Can you work these out from the model? Positions are in its coordinate system, mm. A direction names the side the tool comes from. Coordinates: 2 decimals unless noted, no trailing zeros. Loops run counter-clockwise (first coordinate to the right, second up) from the corner with the lowest first, then second, coordinate; pieces in that order, holes last. Notation, with made-up numbers: (23, 10) -> (62, 10) arc R14 cw to (62, 30) -> close; hole circle Ø9 at (88, 11.5). An arc over 180 degrees is marked (long way). Use one line per item in the form item = value. Start each with the question number.
(1) Imagine slicing it at C-C (x = 12.5). List the corners of the cut face in (y, z) for me, plus the area to 3 significant figures.
(2) I need wall thicknesses on line 1 (X direction, y = 21, z = -35); line 2 (Z direction, x = -29, y = -12.5); line 3 (Z direction, x = -39, y = -20.5). Which ranges of each line are inside material? Lowest first, please. Write a range as [from, to].
(3) Thinking about a two-plate mould opening in X: for faces 6 (the cylindrical face through (-43, -22, -39)), 7 (the cylindrical face through (43, -22, -39)), 8 (the flat face through (35, -21, -20)), which applies, released by +X, released by -X, zero draft, split by the parting line, or undercut?
(4) I'm going to push flat-ended pins straight in: pin 1 (4 mm diameter, centred on x = 8, y = -9.5, fed in from -Z); pin 2 (10 mm diameter, centred on y = -12.5, z = -18, fed in from +X). Where does each tip first touch, or does it pass through?
(5) Imagine slicing it at D-D (z = -3). List the corners of the cut face in (x, y) for me, plus the area to 3 significant figures.
(6) Imagine slicing it at A-A (z = -18.5). List the corners of the cut face in (x, y) for me.
(7) On a 3-axis mill with a long thin cutter (end or side, diameter ignored), from which of +Z, -Z, +X, -X, +Y, -Y can I reach the whole of each face in a straight line? I mean faces 1 (the flat face through (35, 21, -20)), 2 (the flat face through (-39, -20, -20)), 3 (the flat face through (-1, 0, 3)), 4 (the cylindrical face through (-43, 22, -39)), 5 (the flat face through (-1, 0, 0)). Say none if no direction works.
(8) Imagine slicing it at B-B (y = -18). List the corners of the cut face in (x, z) for me, plus the area to 3 significant figures.
```python
from build123d import *

# Parameters (mm, degrees)
SZKIC1_W                    = 90
SZKIC1_H                    = 46
DODANIE_WYCI_GNI_CIE1_DEPTH = 3
SZKIC2_W                    = 10
SZKIC2_H                    = 3
DODANIE_WYCI_GNI_CIE2_DEPTH = 40
SFAZOWANIE1_SIZE            = 5
SFAZOWANIE2_SIZE            = 1
ZAOKR_GLENIE1_R             = 5
SFAZOWANIE1_OF_LUSTRO1_SIZE = 5
SFAZOWANIE2_OF_LUSTRO1_SIZE = 1
ZAOKR_GLENIE1_OF_LUSTRO1_R  = 5
SZKIC3_R                    = 1.75
WYTNIJ_WYCI_GNI_CIE1_DEPTH  = 76.769386958


with BuildPart() as part:
    # Szkic1 → Dodanie-wyciągnięcie1 (new body)
    with BuildSketch(Plane.XY):
        Rectangle(SZKIC1_W, SZKIC1_H)
    extrude(amount=DODANIE_WYCI_GNI_CIE1_DEPTH)

    # Szkic2 → Dodanie-wyciągnięcie2 (add)
    with BuildSketch(Plane(origin=(0, 0, 0), x_dir=(-1, 0, 0), z_dir=(0, 0, -1))):
        with Locations((-40, 21.5)):
            Rectangle(SZKIC2_W, SZKIC2_H)
        with Locations((40, 21.5)):
            Rectangle(SZKIC2_W, SZKIC2_H)
    dodanie_wyci_gni_cie2 = extrude(amount=DODANIE_WYCI_GNI_CIE2_DEPTH)

    # Sfazowanie1
    sfazowanie1_edges = [part.edges().sort_by_distance(p)[0] for p in [
        (35, 21.5, 0),
        (-35, 21.5, 0),
    ]]
    chamfer(sfazowanie1_edges, length=SFAZOWANIE1_SIZE)

    # Sfazowanie2
    sfazowanie2_edges = [part.edges().sort_by_distance(p)[0] for p in [
        (37.5, 20, 0),
        (-37.5, 20, 0),
    ]]
    chamfer(sfazowanie2_edges, length=SFAZOWANIE2_SIZE)

    # Zaokrąglenie1
    zaokr_glenie1_edges = [part.edges().sort_by_distance(p)[0] for p in [
        (35, 21.5, -40),
        (45, 21.5, -40),
        (-35, 21.5, -40),
        (-45, 21.5, -40),
    ]]
    fillet(zaokr_glenie1_edges, radius=ZAOKR_GLENIE1_R - 0.0001)  # a hair under: the kernel refuses the full size

    # Lustro1: Dodanie-wyciągnięcie2 across plane
    add(dodanie_wyci_gni_cie2.mirror(Plane.ZX))

    # Sfazowanie1 of Lustro1
    sfazowanie1_of_lustro1_edges = [part.edges().sort_by_distance(p)[0] for p in [
        (35, -21.5, 0),
        (-35, -21.5, 0),
    ]]
    chamfer(sfazowanie1_of_lustro1_edges, length=SFAZOWANIE1_OF_LUSTRO1_SIZE)

    # Sfazowanie2 of Lustro1
    sfazowanie2_of_lustro1_edges = [part.edges().sort_by_distance(p)[0] for p in [
        (37.5, -20, 0),
        (-37.5, -20, 0),
    ]]
    chamfer(sfazowanie2_of_lustro1_edges, length=SFAZOWANIE2_OF_LUSTRO1_SIZE)

    # Zaokrąglenie1 of Lustro1
    zaokr_glenie1_of_lustro1_edges = [part.edges().sort_by_distance(p)[0] for p in [
        (35, -21.5, -40),
        (45, -21.5, -40),
        (-35, -21.5, -40),
        (-45, -21.5, -40),
    ]]
    fillet(zaokr_glenie1_of_lustro1_edges, radius=ZAOKR_GLENIE1_OF_LUSTRO1_R - 0.0001)  # a hair under: the kernel refuses the full size

    # Szkic3 → Wytnij-wyciągnięcie1 (cut, through all)
    with BuildSketch(Plane(origin=(0, 23, 0), x_dir=(1, 0, 0), z_dir=(0, 1, 0))):
        with Locations(Location((-40, 35, 0), (0, 0, 270))):
            Circle(SZKIC3_R)
        with Locations(Location((40, 35, 0), (0, 0, 270))):
            Circle(SZKIC3_R)
    extrude(amount=-WYTNIJ_WYCI_GNI_CIE1_DEPTH, mode=Mode.SUBTRACT)


solid = part.part
```
Worked out:
q1.outline = (-23, 0) -> (23, 0) -> (23, 3) -> (-23, 3) -> close
q1.area = 138 mm2
q2.line_1 = [-45, -41.75], [-38.25, -35], [35, 38.25], [41.75, 45]
q2.line_2 = [0, 3]
q2.line_3 = [-39.9, -36.44], [-33.56, 3]
q3.face_6 = released by -X
q3.face_7 = released by +X
q3.face_8 = undercut
q4.pin_1 = 0
q4.pin_2 = through
q5.outline = (-45, -23) -> (-33, -23) -> (-33, -20) -> (-45, -20) -> close; (-45, 20) -> (-33, 20) -> (-33, 23) -> (-45, 23) -> close; (33, -23) -> (45, -23) -> (45, -20) -> (33, -20) -> close; (33, 20) -> (45, 20) -> (45, 23) -> (33, 23) -> close
q5.area = 144 mm2
q6.outline = (-45, -23) -> (-35, -23) -> (-35, -20) -> (-45, -20) -> close; (-45, 20) -> (-35, 20) -> (-35, 23) -> (-45, 23) -> close; (35, -23) -> (45, -23) -> (45, -20) -> (35, -20) -> close; (35, 20) -> (45, 20) -> (45, 23) -> (35, 23) -> close
q7.face_1 = -Z, +Y, -Y
q7.face_2 = -Z, +X, -X
q7.face_3 = +Z, +X, -X, +Y, -Y
q7.face_4 = -Z, -X, +Y, -Y
q7.face_5 = -Z
q8.outline = (-45, 0) -> (45, 0) -> (45, 3) -> (-45, 3) -> close
q8.area = 270 mm2
